```python
from build123d import *

# Parameters (mm, degrees)
SKETCH_R     = 13.95
SKETCH_R_2   = 1.5
PAD_DEPTH    = 5
SKETCH001_R  = 13.95
PAD001_DEPTH = 11.7
SKETCH002_R  = 2.5
PAD002_DEPTH = 15
FILLET_R     = 2
FILLET001_R  = 2


with BuildPart() as part:
    # Sketch → Pad (new body)
    with BuildSketch(Plane.XY):
        with Locations((-16.282767, 14.793005)):
            Circle(SKETCH_R)
        with Locations((-25.269844, 17.872364)):
            Circle(SKETCH_R_2, mode=Mode.SUBTRACT)
        with Locations((-18.875912, 7.22494)):
            Circle(SKETCH_R_2, mode=Mode.SUBTRACT)
        with Locations((-7.295691, 11.713645)):
            Circle(SKETCH_R_2, mode=Mode.SUBTRACT)
        with Locations((-13.689622, 22.361069)):
            Circle(SKETCH_R_2, mode=Mode.SUBTRACT)
    extrude(amount=PAD_DEPTH)

    # Sketch001 → Pad001 (new body)
    with BuildSketch(Plane.XY.offset(5)):
        with Locations((-16.282767, 14.793005)):
            Circle(SKETCH001_R)
    extrude(amount=PAD001_DEPTH)

    # Sketch002 → Pad002 (new body)
    with BuildSketch(Plane.XY.offset(16.7)):
        with Locations((-16.282767, 14.793005)):
            Circle(SKETCH002_R)
    extrude(amount=PAD002_DEPTH)

    # Fillet
    fillet_edges = [part.edges().sort_by_distance(p)[0] for p in [
        (-30.232767, 14.793005, 16.7),
    ]]
    fillet(fillet_edges, radius=FILLET_R)

    # Fillet001
    fillet001_edges = [part.edges().sort_by_distance(p)[0] for p in [
        (-30.232767, 14.793005, 0),
    ]]
    fillet(fillet001_edges, radius=FILLET001_R)


solid = part.part
```
Read the model definition and answer for the solid it produces. Units are mm, in the model's axes. A direction names the side the tool comes from. Give positions to 0.01 mm unless a question says otherwise; leave off trailing zeros. Loops run counter-clockwise (first coordinate to the right, second up) from the corner with the lowest first, then second, coordinate; pieces in that order, holes last.
Item 1: For faces 1 (the cylindrical face through (-13.898, 15.544, 24.095)), 2 (the flat face through (-16, 15, 31.7)), 3 (the cylindrical face through (-20.374, 7.291, 2.465)), determine the directions among +Z, -Z, +X, -X, +Y, -Y from which every point of the face is accessible in a straight line to the end or side of a thin tool.
Item 2: Each of these flat-tipped pins is pushed along its axis until it touches: pin 1 Ø2.5 at (x, y) = (-13.69, 22.36) entering from -Z; pin 2 Ø4 at (y, z) = (23.5, 15.5) entering from +X; pin 3 Ø3 at (y, z) = (9.5, 8.5) entering from -X; pin 4 Ø2 at (x, z) = (-5.5, 18) entering from +Y (3 decimals). Where does it stop, or does it pass through?
Item 3: The part is cut by section B-B (z = 10). Write down the section's boundary in (x, y).
Item 4: The part is cut by section C-C (z = 19.5). Write down the section's boundary in (x, y).
Item 5: The mould has two halves that part along Y. Classify faces 4 (the cylindrical face through (-30.22, 15.41, 8.26)), 5 (the flat face through (-16, 15, 0)), 6 (the flat face through (-14, 22, 5)): released by +Y, released by -Y, zero draft, split by the parting line, or undercut.
Item 6: Find the intervals of material crossed by line 1 along Z through (x, y) = (-20.25, 15.25); line 2 along Y through (x, z) = (-10.5, 6); line 3 along Y through (x, z) = (-15.75, 11), in increasing order.
Item 7: The part is cut by section A-A (z = 3). Write down the section's boundary in (x, y), and give its area (3 significant figures).
Taken from the geometry:
1. face 1: +Z
1. face 2: +Z, +X, -X, +Y, -Y
1. face 3: -Z
2. pin 1: stops at z = 5
2. pin 2: stops at x = -4.11
2. pin 3: stops at x = -29.71
2. pin 4: passes through
3. outline: circle Ø27.9 at (-16.28, 14.79)
4. outline: circle Ø5 at (-16.28, 14.79)
5. face 4: split by the parting line
5. face 5: zero draft
5. face 6: undercut
6. line 1: z = 0 to 16.7
6. line 2: y = 2.1 to 27.49
6. line 3: y = 0.85 to 28.73
7. outline: circle Ø27.9 at (-16.28, 14.79); hole circle Ø3 at (-25.27, 17.87); hole circle Ø3 at (-18.88, 7.22); hole circle Ø3 at (-13.69, 22.36); hole circle Ø3 at (-7.3, 11.71)
7. area: 583 mm2
